from build123d import *

# Parameters (mm, degrees)
BASPROSKE_W             = 10
BASPROSKE_H             = 20
TOOTHCUT_DEPTH          = 31
TEETHCUTS_COUNT         = 14
TEETHCUTS_ANGLE         = 334.285714286
BORSKE_R                = 5
BORE_DEPTH              = 50.0000508
BOSS_EXTRU_1_START      = 12.5
ESQUISSE1_R             = 9
ESQUISSE1_R_2           = 5
BOSS_EXTRU_1_DEPTH      = 12.5
ESQUISSE2_R             = 1.980815445
ENL_V_MAT_EXTRU_1_DEPTH = 12.5


with BuildPart() as part:
    # BasProSke → Base-Revolve (revolve)
    with BuildSketch(Plane(origin=(0, 0, 0), x_dir=(1, 0, 0), z_dir=(0, 1, 0)), mode=Mode.PRIVATE) as base_revolve_sk:
        with Locations((5, 10)):
            Rectangle(BASPROSKE_W, BASPROSKE_H)
    revolve(base_revolve_sk.sketch.rotate(Axis((-10, 0, 0), (1, 0, 0)), 180), axis=Axis((-10, 0, 0), (1, 0, 0)))

    # TooCutSke → ToothCut (cut, through all)
    with BuildSketch(Plane(origin=(0, 0, 0), x_dir=(0, 0, -1), z_dir=(1, 0, 0))):
        with BuildLine():
            ThreePointArc((1.558726024, 14.28923543), (0, 14.374), (-1.558726024, 14.28923543))
            ThreePointArc((-1.558726024, 14.28923543), (-2.047638508, 17.217318907), (-3.706114514, 19.679465449))
            ThreePointArc((-3.706114514, 19.679465449), (0, 20.0254), (3.706114514, 19.679465449))
            ThreePointArc((3.706114514, 19.679465449), (2.047638508, 17.217318907), (1.558726024, 14.28923543))
        make_face()
    toothcut = extrude(amount=TOOTHCUT_DEPTH, mode=Mode.SUBTRACT)

    # TeethCuts: ToothCut ×14 about axis
    teethcuts_axis = Axis((-10, 0, 0), (1, 0, 0))
    for i in range(1, TEETHCUTS_COUNT):
        add(toothcut.rotate(teethcuts_axis, i * TEETHCUTS_ANGLE / (TEETHCUTS_COUNT - 1)), mode=Mode.SUBTRACT)

    # BorSke → Bore (cut, symmetric)
    with BuildSketch(Plane(origin=(0, 0, 0), x_dir=(0, 0, -1), z_dir=(1, 0, 0))):
        with Locations(Location((0, 0, 0), (0, 0, 180))):
            Circle(BORSKE_R)
    extrude(amount=BORE_DEPTH, both=True, mode=Mode.SUBTRACT)

    # Esquisse1 → Boss.-Extru.1 (add)
    with BuildSketch(Plane(origin=(10, 0, 0), x_dir=(0, 0, -1), z_dir=(1, 0, 0)).offset(BOSS_EXTRU_1_START)):
        with Locations(Location((0, 0, 0), (0, 0, 180))):
            Circle(ESQUISSE1_R)
        Circle(ESQUISSE1_R_2, mode=Mode.SUBTRACT)
    extrude(amount=-BOSS_EXTRU_1_DEPTH)

    # Esquisse2 → Enlèv. mat.-Extru.1 (cut)
    with BuildSketch(Plane(origin=(0, 0, 0), x_dir=(1, 0, 0), z_dir=(0, 1, 0))):
        with Locations(Location((16.25, 0, 0), (0, 0, 270))):
            Circle(ESQUISSE2_R)
    extrude(amount=-ENL_V_MAT_EXTRU_1_DEPTH, mode=Mode.SUBTRACT)


solid = part.part
Input: part model. Units: mm. Frame: model coordinates. Round coordinates to 2 decimals unless told otherwise and drop trailing zeros. Order: outer loops, then holes, each group sorted by start corner. A loop starts at its lowest first (then second) coordinate and runs counter-clockwise, first axis right, second up. Notation, with made-up numbers: (-29.75, 86.5) - (-0.75, 86.5) arc R29 cw to (-0.75, 111.5) - close; hole circle Ø3 at (52.25, -37). An arc over 180 degrees is marked (long way). Answer as a JSON object with one key per item and string values. Group by question number.
(1) Draft query along Z for faces 1 (the face through (4.93, 17.242, -2.057)), 2 (the face through (5.07, -19.5, -4.44)), 3 (the face through (22.5, 4, 4)), 4 (the face through (5, 16, 12)). Return one class per face: released by +Z, released by -Z, zero draft, split by the parting line, or undercut.
(2) Cut plane A-A (z = 0). Return loops of the section in (x, y), then the cut area to 3 significant figures.
(3) Cut plane B-B (y = 0). Return loops of the section in (x, z), then the cut area to 3 significant figures.
(4) Cut plane C-C (x = 21). Return loops of the section in (y, z), then the cut area to 3 significant figures.
(5) Pin query (flat end, axial travel): P1, Ø5, axis at x = 16.25, z = 0, coming from the -Y side; P2, Ø6, axis at x = 9.5, z = -10, coming from the -Y side; P3, Ø8, axis at y = 0, z = 0, coming from the -X side (3 decimals); P4, Ø6, axis at x = 17.5, y = -7.5, coming from the +Z side. Return the tip coordinate at first contact, or that it passes through.
(6) Cut plane D-D (y = -13). Return loops of the section in (x, z), then the cut area to 3 significant figures.
(7) Material intervals for probe 1 along Y at (x, z) = (9.75, 0); probe 2 along Y at (x, z) = (7.25, -12.5); probe 3 along X at (y, z) = (-7, 0), sorted ascending. Write a range as from..to.
Here are the results:
{
 "1": {"face 1": "undercut", "face 2": "released by -Z", "face 3": "zero draft", "face 4": "released by +Z"},
 "2": {"outline": "(0, -14.37) - (10, -14.37) - (10, -9) - (14.27, -9) - (14.27, -5) - (0, -5) - close; (0, 5) - (22.5, 5) - (22.5, 9) - (10, 9) - (10, 14.37) - (0, 14.37) - close; (18.23, -9) - (22.5, -9) - (22.5, -5) - (18.23, -5) - close", "area": "272 mm^2"},
 "3": {"outline": "(0, -20) - (10, -20) - (10, -9) - (22.5, -9) - (22.5, -5) - (0, -5) - close; (0, 5) - (22.5, 5) - (22.5, 9) - (10, 9) - (10, 20) - (0, 20) - close", "area": "400 mm^2"},
 "4": {"outline": "circle Ø18 at (0, 0); hole circle Ø10 at (0, 0)", "area": "176 mm^2"},
 "5": {"P1": "stops at y = -9", "P2": "stops at y = -16.11", "P3": "passes through", "P4": "stops at z = 7.79"},
 "6": {"outline": "(0, -12.52) - (10, -12.52) - (10, -8.01) - (0, -8.01) - close; (0, -6.13) - (10, -6.13) - (10, 6.13) - (0, 6.13) - close; (0, 8.01) - (10, 8.01) - (10, 12.52) - (0, 12.52) - close", "area": "213 mm^2"},
 "7": {"probe 1": "y = -14.37..-5, 5..14.37", "probe 2": "y = -15.61..-12.96, -7.98..7.98, 12.96..15.61", "probe 3": "x = 0..14.27, 18.23..22.5"}
}
